Autodesk Fusion 360 part; units mm, degrees
sketch "スケッチ1" plane through (0, 0, 0) normal (0, 0, 1) x (1, 0, 0)
  line L0 (3, 1.7321) -> (0, 3.4641)
  line L1 (0, 3.4641) -> (-3, 1.7321)
  line L2 (-3, 1.7321) -> (-3, -1.7321)
  line L3 (-3, -1.7321) -> (0, -3.4641)
  line L4 (0, -3.4641) -> (3, -1.7321)
  line L5 (3, -1.7321) -> (3, 1.7321)
  circle A0 centre (0, 0) radius 1.5
extrude "押し出し1" add sketch "スケッチ1" along normal blind 35
sketch "スケッチ2" plane through (0, 0, 35) normal (0, 0, 1) x (-1, 0, 0)
  circle A0 centre (0, 0) radius 1.5
  line L0 (-3, 1.7321) -> (-3, -1.7321)
  line L1 (-3, -1.7321) -> (0, -3.4641)
  line L2 (0, -3.4641) -> (3, -1.7321)
  line L3 (3, -1.7321) -> (3, 1.7321)
  line L4 (3, 1.7321) -> (0, 3.4641)
  line L5 (0, 3.4641) -> (-3, 1.7321)
  line L6 (-3.5, 0) -> (-1.75, -3.0311)
  line L7 (-1.75, -3.0311) -> (1.75, -3.0311)
  line L8 (1.75, -3.0311) -> (3.5, 0)
  line L9 (3.5, 0) -> (1.75, 3.0311)
  line L10 (1.75, 3.0311) -> (-1.75, 3.0311)
  line L11 (-1.75, 3.0311) -> (-3.5, 0)
extrude "押し出し2" add sketch "スケッチ2" along normal blind 4 contours L0 L1 L2 L3 L4 L5 L6 L7 L8 L9 L10 L11 | L0 L6 L11 | L5 L10 L11 | L1 L6 L7 | L4 L9 L10 | L2 L7 L8 | L3 L8 L9
extrude "押し出し3" cut 6 faces at (0, -3.1754, 35) (2.75, -1.5877, 35) (-2.75, -1.5877, 35) (-2.75, 1.5877, 35) (0, 3.1754, 35) (2.75, 1.5877, 35) along direction (0, 0, -1) blind 40
extrude "押し出し4" add 6 faces at (1.5833, 2.7424, 35) (3.1667, 0, 35) (-1.5833, 2.7424, 35) (1.5833, -2.7424, 35) (-1.5833, -2.7424, 35) (-3.1667, 0, 35) along direction (0, 0, -1) blind 35
extrude "押し出し5" cut 1 faces at (2.2005, 1.2273, 39) along direction (0, 0, -1) blind 4
extrude "押し出し6" add 1 faces at (0.0374, 2.5193, 35) along direction (0, 0, 1) blind 10
extrude "押し出し7" add 1 faces at (0.0374, 2.5193, 45) along direction (0, 0, 1) blind 40
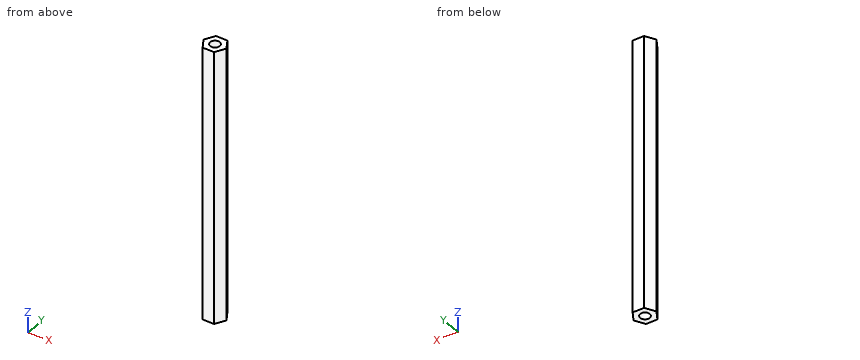
Check sheet for the modelled part. Datum: model origin and axes. Units: mm. Coordinates: 2 decimals unless noted, no trailing zeros. Write each loop counter-clockwise with the first axis right and the second up, starting at its lowest first coordinate (ties: lowest second). Pieces come first, ordered by that corner, then holes. Notation, with made-up numbers: (85, 58) -> (117, 58) arc R36 cw to (117, 95) -> close; hole circle Ø9 at (8.25, 55). An arc over 180 degrees is marked (long way). Use a Markdown table: item, result.
1. Scan lines: line 1 along Y through (x, z) = (0, 45.5); line 2 along X through (y, z) = (3, 74.5); line 3 along Y through (x, z) = (-0.5, 48). Record each from-to range of solid material in increasing order.
Reported:
| item | result |
|---|---|
| line 1 | y = -3.03 to -1.5, 1.5 to 3.03 |
| line 2 | x = -1.77 to 1.77 |
| line 3 | y = -3.03 to -1.41, 1.41 to 3.03 |
2. Go/stop test with a flat-tipped pin: pin 1 Ø1 at (y, z) = (-1, 36.5) entering from -X. Record where the tip stops, or that it passes through.
Reported:
| item | result |
|---|---|
| pin 1 | stops at x = -3.21 |
3. Sectioned sample at A-A (x = 0). Enter the section's corners in (y, z), plus the area to 3 significant figures.
Reported:
| item | result |
|---|---|
| outline | (-3.03, 0) -> (-1.5, 0) -> (-1.5, 85) -> (-3.03, 85) -> close; (1.5, 0) -> (3.03, 0) -> (3.03, 85) -> (1.5, 85) -> close |
| area | 260 mm2 |
4. Sectioned sample at B-B (z = 8). Enter the section's corners in (x, y).
Reported:
| item | result |
|---|---|
| outline | (-3.5, 0) -> (-1.75, -3.03) -> (1.75, -3.03) -> (3.5, 0) -> (1.75, 3.03) -> (-1.75, 3.03) -> close; hole circle Ø3 at (0, 0) |
5. Sectioned sample at C-C (y = 2.25). Enter the section's corners in (x, z).
Reported:
| item | result |
|---|---|
| outline | (-2.2, 0) -> (2.2, 0) -> (2.2, 85) -> (-2.2, 85) -> close |
